Verification items for the finished model (mm, model axes). A direction names the side the tool comes from. Round coordinates to 2 decimals unless told otherwise and drop trailing zeros. Loops run counter-clockwise (first coordinate to the right, second up) from the corner with the lowest first, then second, coordinate; pieces in that order, holes last. Notation, with made-up numbers: (26.25, 49.25) - (82.25, 49.25) arc R29 ccw to (82.25, 75.25) - close; hole circle Ø10 at (16, -34.75). An arc over 180 degrees is marked (long way). Use a Markdown table: item, result. Add a question column.
```python
from build123d import *

# Parameters (mm, degrees)
SKETCH2_R           = 5
BOSS_EXTRUDE1_DEPTH = 8
SKETCH3_W           = 15
SKETCH3_H           = 15
BOSS_EXTRUDE2_DEPTH = 12
SKETCH4_R           = 4
CUT_EXTRUDE1_DEPTH  = 1
FILLET1_R           = 1.5


with BuildPart() as part:
    # Sketch2 → Boss-Extrude1 (new body)
    with BuildSketch(Plane.ZY.offset(36.137829577)):
        with Locations((-25, -31.600577771)):
            Circle(SKETCH2_R)
    extrude(amount=BOSS_EXTRUDE1_DEPTH)

    # Sketch3 → Boss-Extrude2 (add)
    with BuildSketch(Plane(origin=(-36.137829577, 0, 0), x_dir=(0, 0, -1), z_dir=(1, 0, 0))):
        with Locations((25, -31.600577771)):
            Rectangle(SKETCH3_W, SKETCH3_H)
    extrude(amount=BOSS_EXTRUDE2_DEPTH)

    # Sketch4 → Cut-Extrude1 (cut)
    with BuildSketch(Plane.ZY.offset(44.137829577)):
        with Locations((-25, -31.600577771)):
            Circle(SKETCH4_R)
    extrude(amount=-CUT_EXTRUDE1_DEPTH, mode=Mode.SUBTRACT)

    # Fillet1
    fillet1_edges = [part.edges().sort_by_distance(p)[0] for p in [
        (-30.137829577, -24.100577771, -17.5),
        (-30.137829577, -24.100577771, -32.5),
        (-30.137829577, -39.100577771, -17.5),
        (-30.137829577, -39.100577771, -32.5),
    ]]
    fillet(fillet1_edges, radius=FILLET1_R)


solid = part.part
```
Q1. Section check A-A on z = -25. Record the cut outline in (x, y).
Q2. Release check for a two-part mould opening along Z. For faces 1 (the face through (-43.6, -34, -28.2)), 2 (the face through (-24.138, -31, -25)), 3 (the face through (-30.05, -24.53, -32.05)) record: +Z half, -Z half, draft (parallel to the pull), parting line (faces both ways), or undercut.
Q3. Section check B-B on y = -32.75. Record the cut outline in (x, z), plus the area to 3 significant figures.
Q4. Set-up check for faces 4 (the face through (-44.138, -33, -29)), 5 (the face through (-43.138, -32, -25)): record each of +Z, -Z, +X, -X, +Y, -Y from which the full face is reachable in a straight line by a thin tool's end or side.
Q5. Go/stop test with flat-tipped pins: pin 1 Ø2 at (y, z) = (-32.5, -21.5) entering from -X; pin 2 Ø1 at (x, y) = (-42, -31) entering from +Z. Record where each tip stops, or that it passes through.
Q6. Section check D-D on x = -39.5. Record the cut outline in (y, z), plus the area to 3 significant figures.
Q7. Thickness scan on line 1 along Y through (x, z) = (-43.6, -25); line 2 along X through (y, z) = (-36, -22.5); line 3 along X through (y, z) = (-33.75, -26.5). Record the ranges inside material, lowest first.
Q8. Section check C-C on y = -37. Record the cut outline in (x, z), plus the area to 3 significant figures.
Determined:
| question | item | result |
|---|---|---|
| 1 | outline | (-44.14, -36.6) - (-36.14, -36.6) - (-36.14, -39.1) - (-24.14, -39.1) - (-24.14, -24.1) - (-36.14, -24.1) - (-36.14, -26.6) - (-44.14, -26.6) - (-44.14, -27.6) - (-43.14, -27.6) - (-43.14, -35.6) - (-44.14, -35.6) - close |
| 2 | face 1 | undercut |
| 2 | face 2 | draft |
| 2 | face 3 | -Z half |
| 3 | outline | (-44.14, -29.87) - (-36.14, -29.87) - (-36.14, -32.5) - (-24.14, -32.5) - (-24.14, -17.5) - (-36.14, -17.5) - (-36.14, -20.13) - (-44.14, -20.13) - (-44.14, -21.17) - (-43.14, -21.17) - (-43.14, -28.83) - (-44.14, -28.83) - close |
| 3 | area | 250 mm² |
| 4 | face 4 | +Z, -Z, -X, +Y, -Y |
| 4 | face 5 | -X |
| 5 | pin 1 | stops at x = -44.14 |
| 5 | pin 2 | stops at z = -20 |
| 6 | outline | circle Ø10 at (-31.6, -25) |
| 6 | area | 78.5 mm² |
| 7 | line 1 | y = -36.6 to -35.6, -27.6 to -26.6 |
| 7 | line 2 | x = -36.14 to -24.14 |
| 7 | line 3 | x = -43.14 to -24.14 |
| 8 | outline | (-36.14, -32.5) - (-24.14, -32.5) - (-24.14, -17.5) - (-36.14, -17.5) - close |
| 8 | area | 180 mm² |
